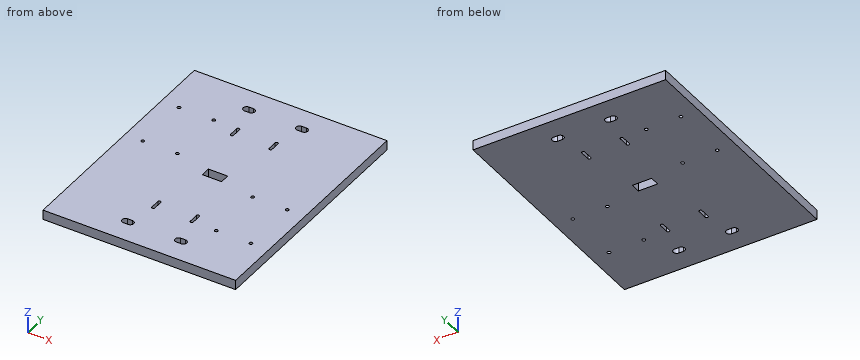
from build123d import *

# Parameters (mm, degrees)
ESQUISSE2_W             = 200
ESQUISSE2_H             = 250
BOSS_EXTRU_1_DEPTH      = 10
ESQUISSE7_W             = 20
ESQUISSE7_H             = 10
ENL_V_MAT_EXTRU_2_DEPTH = 10
ENL_V_MAT_EXTRU_3_DEPTH = 10
ENL_V_MAT_EXTRU_4_DEPTH = 10
D_GAGEMENT_M31_D        = 3.4


with BuildPart() as part:
    # Esquisse2 → Boss.-Extru.1 (new body)
    with BuildSketch(Plane.XY):
        with Locations((100, -125)):
            Rectangle(ESQUISSE2_W, ESQUISSE2_H)
    extrude(amount=BOSS_EXTRU_1_DEPTH)

    # Esquisse7 → Enlèv. mat.-Extru.2 (cut)
    with BuildSketch(Plane(origin=(0, 0, 0), x_dir=(-1, 0, 0), z_dir=(0, 0, -1))):
        with Locations((-100, -125)):
            Rectangle(ESQUISSE7_W, ESQUISSE7_H)
    extrude(amount=-ENL_V_MAT_EXTRU_2_DEPTH, mode=Mode.SUBTRACT)

    # Esquisse10 → Enlèv. mat.-Extru.3 (cut)
    with BuildSketch(Plane(origin=(0, 0, 0), x_dir=(-1, 0, 0), z_dir=(0, 0, -1))):
        with BuildLine():
            Line((-70, -28.5), (-75, -28.5))
            ThreePointArc((-75, -28.5), (-78.5, -25), (-75, -21.5))
            Line((-75, -21.5), (-70, -21.5))
            ThreePointArc((-70, -21.5), (-66.5, -25), (-70, -28.5))
        make_face()
        with BuildLine():
            Line((-70, -228.5), (-75, -228.5))
            ThreePointArc((-75, -228.5), (-78.5, -225), (-75, -221.5))
            Line((-75, -221.5), (-70, -221.5))
            ThreePointArc((-70, -221.5), (-66.5, -225), (-70, -228.5))
        make_face()
        with BuildLine():
            Line((-130, -221.5), (-125, -221.5))
            ThreePointArc((-125, -221.5), (-121.5, -225), (-125, -228.5))
            Line((-125, -228.5), (-130, -228.5))
            ThreePointArc((-130, -228.5), (-133.5, -225), (-130, -221.5))
        make_face()
        with BuildLine():
            Line((-130, -21.5), (-125, -21.5))
            ThreePointArc((-125, -21.5), (-121.5, -25), (-125, -28.5))
            Line((-125, -28.5), (-130, -28.5))
            ThreePointArc((-130, -28.5), (-133.5, -25), (-130, -21.5))
        make_face()
    extrude(amount=-ENL_V_MAT_EXTRU_3_DEPTH, mode=Mode.SUBTRACT)

    # Esquisse11 → Enlèv. mat.-Extru.4 (cut)
    with BuildSketch(Plane(origin=(0, 0, 0), x_dir=(-1, 0, 0), z_dir=(0, 0, -1))):
        with BuildLine():
            Line((-78.5, -55), (-78.5, -65))
            ThreePointArc((-78.5, -65), (-80, -66.5), (-81.5, -65))
            Line((-81.5, -65), (-81.5, -55))
            ThreePointArc((-81.5, -55), (-80, -53.5), (-78.5, -55))
        make_face()
        with BuildLine():
            Line((-118.5, -55), (-118.5, -65))
            ThreePointArc((-118.5, -65), (-120, -66.5), (-121.5, -65))
            Line((-121.5, -65), (-121.5, -55))
            ThreePointArc((-121.5, -55), (-120, -53.5), (-118.5, -55))
        make_face()
        with BuildLine():
            Line((-121.5, -195), (-121.5, -185))
            ThreePointArc((-121.5, -185), (-120, -183.5), (-118.5, -185))
            Line((-118.5, -185), (-118.5, -195))
            ThreePointArc((-118.5, -195), (-120, -196.5), (-121.5, -195))
        make_face()
        with BuildLine():
            Line((-81.5, -195), (-81.5, -185))
            ThreePointArc((-81.5, -185), (-80, -183.5), (-78.5, -185))
            Line((-78.5, -185), (-78.5, -195))
            ThreePointArc((-78.5, -195), (-80, -196.5), (-81.5, -195))
        make_face()
    extrude(amount=-ENL_V_MAT_EXTRU_4_DEPTH, mode=Mode.SUBTRACT)

    # Dégagement M31 (through all)
    with Locations(Plane.XY.offset(10)):
        with Locations((18.5, -54.7), (54.5, -54.7), (18.545923706, -114.7), (54.5, -114.7), (145.5, -135.3), (181.5, -135.3), (145.5, -195.3), (181.5, -195.3)):
            Hole(D_GAGEMENT_M31_D / 2)


solid = part.part
The listing builds one solid part. Answer for the finished solid, in the listing's coordinates (mm). Coordinates: 2 decimals unless noted, no trailing zeros. Write each loop counter-clockwise with the first axis right and the second up, starting at its lowest first coordinate (ties: lowest second). Pieces come first, ordered by that corner, then holes. Notation, with made-up numbers: M 84,20 L 135,20 A14 cw 135,26 Z; hole C 31.25,22.5 d7. An arc over 180 degrees is marked long. Put each result on its own line as item: value. Start each with the question number.
1. A cutting plane is placed at A-A on y = -25. Write down the section's boundary in (x, z).
2. Consider line 1 (X direction, y = -114.7, z = 7.25); line 2 (X direction, y = -186.5, z = 8.75); line 3 (X direction, y = -195.3, z = 7.25). Determine where each line is inside the solid, lowest interval first. Write a range as from..to.
3. A flat-ended cylindrical pin translates along its axis: P1, Ø4, axis at x = 145.5, y = -135.3, coming from the +Z side. Find the tip coordinate at first contact, or state that the pin passes through.
Resolved:
1. outline: M 0,0 L 66.5,0 L 66.5,10 L 0,10 Z; M 78.5,0 L 121.5,0 L 121.5,10 L 78.5,10 Z; M 133.5,0 L 200,0 L 200,10 L 133.5,10 Z
2. line 1: x = 0..16.85, 20.25..52.8, 56.2..200
2. line 2: x = 0..78.5, 81.5..118.5, 121.5..200
2. line 3: x = 0..78.53, 81.47..118.53, 121.47..143.8, 147.2..179.8, 183.2..200
3. P1: stops at z = 10
